Geometry check sheet. Reference: the model listing, model coordinates, mm. Face numbers are marked on the shaded views. A direction names the side the tool comes from. Round coordinates to 2 decimals unless told otherwise and drop trailing zeros. Order: outer loops, then holes, each group sorted by start corner. A loop starts at its lowest first (then second) coordinate and runs counter-clockwise, first axis right, second up. Notation, with made-up numbers: (67, 76.25) - (93, 76.25) arc R7 ccw to (93, 88.25) - close; hole circle Ø1 at (46, -1). An arc over 180 degrees is marked (long way). Write each question's results on one line, items separated by ' | '.
```python
from build123d import *

# Parameters (mm, degrees)
SKETCH_1_R           = 2
EXTRUDE_1_DEPTH      = 1.5
SKETCH_2_W           = 3
SKETCH_2_H           = 50
SKETCH_2_H_2         = 40
EXTRUDE_3_DEPTH      = 8
EXTRUDE_4_DEPTH      = 2
SKETCH_4_W           = 71.000000198
SKETCH_4_H           = 50
CUT_EXTRUDE_1_DEPTH  = 128.300477144
CUT_EXTRUDE_3_DEPTH  = 128.427082997
SKETCH_11_W          = 18.075
SKETCH_11_H          = 14.197672296
CUT_EXTRUDE_4_DEPTH  = 128.300477144
HOLE_WIZARD_M2_5_1_D = 2.55


with BuildPart() as part:
    # 草圖1 → 填料-伸長1 (new body)
    with BuildSketch(Plane.XY):
        with BuildLine():
            Line((-78.58357781, -93.341907955), (16.519190028, -93.341907955))
            Line((16.519190028, -93.341907955), (23.019189929, -93.341907955))
            ThreePointArc((23.019189929, -93.341907955), (23.72629671, -93.049014736), (24.019189929, -92.341907955))
            Line((24.019189929, -92.341907955), (24.019189929, -26.916101175))
            ThreePointArc((24.019189929, -26.916101175), (23.715868617, -26.228364762), (23.019189929, -25.946187519))
            Line((23.019189929, -25.946187519), (16.519190028, -25.946187519))
            ThreePointArc((16.519190028, -25.946187519), (11.569442559, -23.895934988), (9.519190028, -18.946187519))
            Line((9.519190028, -18.946187519), (9.519190028, -5.659090909))
            ThreePointArc((9.519190028, -5.659090909), (9.226296809, -4.951984128), (8.519190028, -4.659090909))
            Line((8.519190028, -4.659090909), (-70.48081017, -4.659090909))
            ThreePointArc((-70.48081017, -4.659090909), (-71.187916951, -4.951984128), (-71.48081017, -5.659090909))
            Line((-71.48081017, -5.659090909), (-71.48081017, -18.946187519))
            ThreePointArc((-71.48081017, -18.946187519), (-73.531062702, -23.895934988), (-78.48081017, -25.946187519))
            Line((-78.48081017, -25.946187519), (-84.980810071, -25.946187519))
            ThreePointArc((-84.980810071, -25.946187519), (-85.687916853, -26.239080738), (-85.980810071, -26.946187519))
            Line((-85.980810071, -26.946187519), (-85.980810071, -92.341911374))
            ThreePointArc((-85.980810071, -92.341911374), (-85.688840793, -93.048093006), (-84.983425077, -93.341907955))
            Line((-84.983425077, -93.341907955), (-78.58357781, -93.341907955))
        make_face()
        with Locations((-79.980810071, -31.644049447)):
            Circle(SKETCH_1_R, mode=Mode.SUBTRACT)
        with Locations((18.019189929, -31.644049447)):
            Circle(SKETCH_1_R, mode=Mode.SUBTRACT)
        with Locations((18.019189929, -87.644049447)):
            Circle(SKETCH_1_R, mode=Mode.SUBTRACT)
        with Locations((-79.980810071, -87.644049447)):
            Circle(SKETCH_1_R, mode=Mode.SUBTRACT)
    extrude(amount=EXTRUDE_1_DEPTH)

    # 草圖2 → 填料-伸長3 (add)
    with BuildSketch(Plane.XY.offset(1.5)):
        with Locations((-67.98081017, -32.85713984)):
            Rectangle(SKETCH_2_W, SKETCH_2_H)
        with Locations((6.019190028, -27.85713984)):
            Rectangle(SKETCH_2_W, SKETCH_2_H_2)
    extrude(amount=EXTRUDE_3_DEPTH)

    # 草圖3 → 填料-伸長4 (add)
    with BuildSketch(Plane.XY.offset(9.5)):
        Polygon((-69.48081017, -17.828011501), (7.519190028, -17.828011501), (7.519190028, -47.85713984), (-8.225095928, -47.85713984), (-8.225095928, -57.85713984), (-69.48081017, -57.85713984), align=None)
    extrude(amount=EXTRUDE_4_DEPTH)

    # 草圖4 → 除料-伸長1 (cut, through all)
    with BuildSketch(Plane.XY.offset(1.5)):
        with Locations((-30.980810071, -32.85713984)):
            Rectangle(SKETCH_4_W, SKETCH_4_H)
    extrude(amount=-CUT_EXTRUDE_1_DEPTH, mode=Mode.SUBTRACT)

    # 草圖7 → 除料-伸長3 (cut, through all)
    with BuildSketch(Plane.XY.offset(11.5)):
        Polygon((-16.225095928, -49.85713984), (-16.225095928, -39.85713984), (-0.480809972, -39.85713984), (-0.480809972, -25.828011501), (-61.48081017, -25.828011501), (-61.48081017, -49.85713984), align=None)
    extrude(amount=-CUT_EXTRUDE_3_DEPTH, mode=Mode.SUBTRACT)

    # 草圖11 → 除料-伸長4 (cut, through all)
    with BuildSketch(Plane.XY.offset(1.5)):
        with Locations((2.751904461, -86.243071807)):
            Rectangle(SKETCH_11_W, SKETCH_11_H)
    extrude(amount=-CUT_EXTRUDE_4_DEPTH, mode=Mode.SUBTRACT)

    # M2.5 螺旋的螺孔鑽1 (through all)
    with Locations(Plane(origin=(0, 0, 0), x_dir=(1, 0, 0), z_dir=(0, 0, -1))):
        with Locations((-64.13081017, 20.20713984), (-0.33081017, 20.20713984), (10.589404461, 70.471994299), (-5.010595539, 70.471994299), (-10.419668394, 72.571170345), (-38.419668394, 72.571170345), (-42.919668394, 69.961668418), (-70.919668394, 69.961668418)):
            Hole(HOLE_WIZARD_M2_5_1_D / 2)


solid = part.part
```
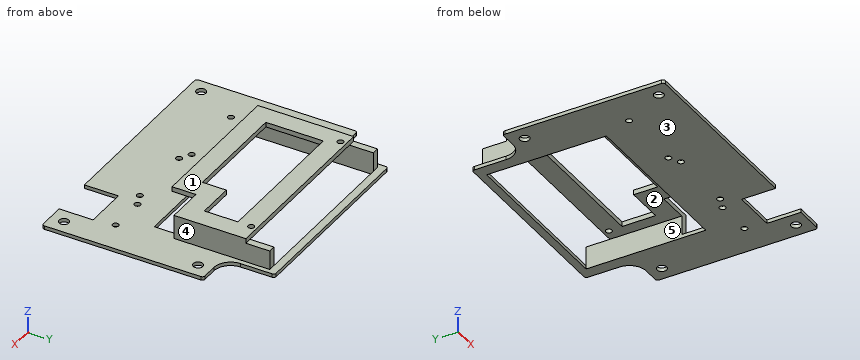
(1) Material ranges on line 1 (X direction, y = -18, z = 8); line 2 (X direction, y = -31, z = 10.75); line 3 (Z direction, x = -42, y = -71.5), recorded low to high.
Answers follow:
line 1: -69.48 to -66.48, 4.52 to 7.52 | line 2: -69.48 to -61.48, -0.48 to 7.52 | line 3: 0 to 1.5
(2) Depth check by flat-ended pin: pin 1 Ø0.8 at (x, z) = (0.5, 0.5) entering from -Y; pin 2 Ø0.9 at (x, y) = (5.5, -10.5) entering from +Z; pin 3 Ø3 at (y, z) = (-18.5, 6.5) entering from +X; pin 4 Ø1.5 at (x, y) = (-42.92, -69.96) entering from +Z. Enter the tip coordinate at first touch or a pass-through.
Answers follow:
pin 1: y = -79.14 | pin 2: z = 9.5 | pin 3: x = 7.52 | pin 4: through
(3) Section check B-B (z = 4.5). Record the cut outline in (x, y).
Answers follow:
outline: (-69.48, -57.86) - (-66.48, -57.86) - (-66.48, -7.86) - (-69.48, -7.86) - close; (4.52, -47.86) - (7.52, -47.86) - (7.52, -7.86) - (4.52, -7.86) - close
(4) Section check C-C (x = -22.5). Record the cut outline in (y, z).
Answers follow:
outline: (-93.34, 0) - (-57.86, 0) - (-57.86, 1.5) - (-93.34, 1.5) - close; (-57.86, 9.5) - (-49.86, 9.5) - (-49.86, 11.5) - (-57.86, 11.5) - close; (-25.83, 9.5) - (-17.83, 9.5) - (-17.83, 11.5) - (-25.83, 11.5) - close; (-7.86, 0) - (-4.66, 0) - (-4.66, 1.5) - (-7.86, 1.5) - close
(5) Access from +Z, -Z, +X, -X, +Y, -Y to the whole of each face (thin tool, end or side, straight path). Record for the marked faces 1 and 2.
Answers follow:
face 1: +Z, +X, -X, +Y, -Y | face 2: -Z, +Y, -Y
(6) Section check A-A (y = -37). Record the cut outline in (x, z).
Answers follow:
outline: (-85.98, 0) - (-66.48, 0) - (-66.48, 9.5) - (-61.48, 9.5) - (-61.48, 11.5) - (-69.48, 11.5) - (-69.48, 1.5) - (-85.98, 1.5) - close; (-0.48, 9.5) - (4.52, 9.5) - (4.52, 0) - (24.02, 0) - (24.02, 1.5) - (7.52, 1.5) - (7.52, 11.5) - (-0.48, 11.5) - close
(7) Section check D-D (y = -13). Record the cut outline in (x, z).
Answers follow:
outline: (-71.48, 0) - (-66.48, 0) - (-66.48, 9.5) - (-69.48, 9.5) - (-69.48, 1.5) - (-71.48, 1.5) - close; (4.52, 0) - (9.52, 0) - (9.52, 1.5) - (7.52, 1.5) - (7.52, 9.5) - (4.52, 9.5) - close
(8) Draft check along X on the marked faces 3, 4 and 5. Enter one of: released by +X, released by -X, zero draft, split by the parting line, or undercut.
Answers follow:
face 3: zero draft | face 4: released by +X | face 5: undercut
